Could you check a few things on this model? Use its own coordinates, in mm. Coordinates: 2 decimals unless noted, no trailing zeros. Write each loop counter-clockwise with the first axis right and the second up, starting at its lowest first coordinate (ties: lowest second). Pieces come first, ordered by that corner, then holes.
Item 1: For P1, Ø12, axis at x = -31.75, y = -43.18, coming from the -Z side; P2, Ø21.5, axis at x = 31.75, y = 25.4, coming from the -Z side, each with a flat end and sliding along its axis, tell me the tip position at first contact or that it passes through.
Item 2: I want a section at A-A on y = 25.4. Please give me the cut outline in (x, z).
Item 3: If I drill on probe 1 along Y at (x, z) = (-31.75, 3.5); probe 2 along X at (y, z) = (-48, 1.75); probe 3 along Y at (x, z) = (67, 6), over which ranges is the centre line in solid material (lowest first)?
Item 4: I want a section at B-B on x = 31.75. Please give me the cut outline in (y, z), then the cut area to 3 significant figures.
Item 5: I want a section at C-C on z = 2.5. Please give me the cut outline in (x, y), then the cut area to 3 significant figures.
Item 6: Thinking about a two-plate mould opening in Y: for faces 1 (the flat face through (-1, -69.85, 3)), 2 (the flat face through (-1, 1, 6.35)), 3 (the flat face through (-1, 69.85, 3)), 4 (the cylindrical face through (38.49, -42.88, 3.13)), which applies, +Y half, -Y half, draft (parallel to the pull), parting line (faces both ways), or undercut?
from build123d import *

# Parameters (mm, degrees)
SKETCH1_W               = 152.4
SKETCH1_H               = 139.7
EXTRUDE1_DEPTH          = 6.35
CHAMFER1_SIZE           = 0.762
F_1_2_CLEARANCE_HOLE1_D = 13.49248


with BuildPart() as part:
    # Sketch1 → Extrude1 (new body)
    with BuildSketch(Plane.XY):
        Rectangle(SKETCH1_W, SKETCH1_H)
    extrude(amount=EXTRUDE1_DEPTH)

    # Chamfer1
    chamfer1_edges = [part.edges().sort_by_distance(p)[0] for p in [
        (76.2, 0, 6.35),
        (0, 69.85, 6.35),
        (-76.2, 0, 6.35),
        (0, 69.85, 0),
        (76.2, 0, 0),
        (0, -69.85, 0),
        (-76.2, 0, 0),
        (0, -69.85, 6.35),
    ]]
    chamfer(chamfer1_edges, length=CHAMFER1_SIZE)

    # 1/2 Clearance Hole1 (through all)
    with Locations(Plane.XY.offset(6.35)):
        with Locations((-31.75, 25.4), (31.75, 25.4), (-31.75, -43.18), (31.75, -43.18)):
            Hole(F_1_2_CLEARANCE_HOLE1_D / 2)


solid = part.part
Response values:
1. P1: passes through
1. P2: stops at z = 0
2. outline: (-76.2, 0.76) - (-75.44, 0) - (-38.5, 0) - (-38.5, 6.35) - (-75.44, 6.35) - (-76.2, 5.59) - close; (-25, 0) - (25, 0) - (25, 6.35) - (-25, 6.35) - close; (38.5, 0) - (75.44, 0) - (76.2, 0.76) - (76.2, 5.59) - (75.44, 6.35) - (38.5, 6.35) - close
3. probe 1: y = -69.85 to -49.93, -36.43 to 18.65, 32.15 to 69.85
3. probe 2: x = -76.2 to -36.47, -27.03 to 27.03, 36.47 to 76.2
3. probe 3: y = -69.44 to 69.44
4. outline: (-69.85, 0.76) - (-69.09, 0) - (-49.93, 0) - (-49.93, 6.35) - (-69.09, 6.35) - (-69.85, 5.59) - close; (-36.43, 0) - (18.65, 0) - (18.65, 6.35) - (-36.43, 6.35) - close; (32.15, 0) - (69.09, 0) - (69.85, 0.76) - (69.85, 5.59) - (69.09, 6.35) - (32.15, 6.35) - close
4. area: 715 mm2
5. outline: (-76.2, -69.85) - (76.2, -69.85) - (76.2, 69.85) - (-76.2, 69.85) - close; hole circle Ø13.49 at (-31.75, -43.18); hole circle Ø13.49 at (-31.75, 25.4); hole circle Ø13.49 at (31.75, -43.18); hole circle Ø13.49 at (31.75, 25.4)
5. area: 20,700 mm2
6. face 1: -Y half
6. face 2: draft
6. face 3: +Y half
6. face 4: undercut
